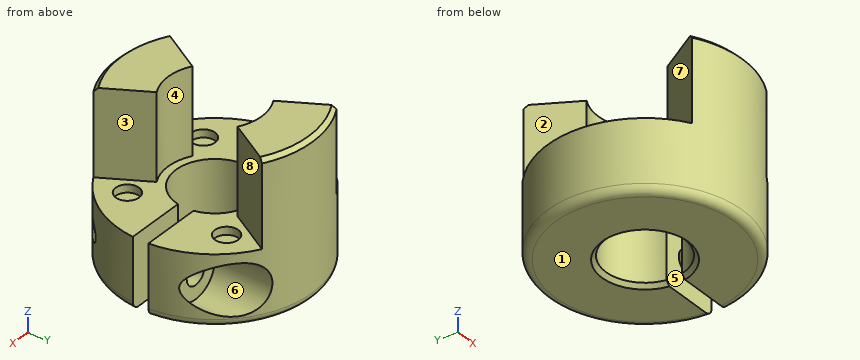
from build123d import *

# Parameters (mm, degrees)
ESBO_O1_R                 = 12.5
RESSALTO_EXTRUS_O1_DEPTH  = 20
CORTE_EXTRUS_O3_DEPTH     = 11
ESBO_O3_R                 = 5
CORTE_EXTRUS_O4_DEPTH     = 21
ESBO_O6_W                 = 12
ESBO_O6_H                 = 2
CORTE_EXTRUS_O5_DEPTH     = 10
CORTE_EXTRUS_O6_START     = -3
ESBO_O7_R                 = 3.25
CORTE_EXTRUS_O6_DEPTH     = 9.5
FURO_ROSCADO_DE_M3X0_51_D = 2.5
FILETE1_R                 = 1
ESBO_O10_R                = 1.5
CORTE_EXTRUS_O7_DEPTH     = 1
CHANFRO1_SIZE             = 0.5
CORTE_EXTRUS_O8_REACH     = 18.5
ESBO_O11_R                = 1.5
ESBO_O12_R                = 6
CORTE_EXTRUS_O9_DEPTH     = 11
PADR_OCIRCULAR1_COUNT     = 4
CHANFRO2_SIZE             = 0.5


with BuildPart() as part:
    # Esboço1 → Ressalto-extrusão1 (new body)
    with BuildSketch(Plane.XY):
        Circle(ESBO_O1_R)
    extrude(amount=RESSALTO_EXTRUS_O1_DEPTH)

    # Esboço2 → Corte-extrusão3 (cut)
    with BuildSketch(Plane.XY.offset(20)):
        with BuildLine():
            Line((0, 0), (6.25, 10.825317547))
            ThreePointArc((6.25, 10.825317547), (12.5, 0), (6.25, -10.825317547))
            Line((6.25, -10.825317547), (0, 0))
        make_face()
    corte_extrus_o3 = extrude(amount=-CORTE_EXTRUS_O3_DEPTH, mode=Mode.SUBTRACT)

    # Esboço3 → Corte-extrusão4 (cut, through all)
    with BuildSketch(Plane(origin=(0, 0, 0), x_dir=(-1, 0, 0), z_dir=(0, 0, -1))):
        Circle(ESBO_O3_R)
    extrude(amount=-CORTE_EXTRUS_O4_DEPTH, mode=Mode.SUBTRACT)

    # Espelhar1: Corte-extrusão3 across plane
    add(corte_extrus_o3.mirror(Plane(origin=(0, 0, 0), x_dir=(0, 0, 1), z_dir=(1, 0, 0))), mode=Mode.SUBTRACT)

    # Esboço6 → Corte-extrusão5 (cut, through all)
    with BuildSketch(Plane.XY.offset(9)):
        with Locations((7, 0)):
            Rectangle(ESBO_O6_W, ESBO_O6_H)
    extrude(amount=-CORTE_EXTRUS_O5_DEPTH, mode=Mode.SUBTRACT)

    # Esboço7 → Corte-extrusão6 (cut, through all)
    with BuildSketch(Plane.XZ.offset(-1).offset(CORTE_EXTRUS_O6_START)):
        with Locations((8.459935794, 4.5)):
            Circle(ESBO_O7_R)
    extrude(amount=-CORTE_EXTRUS_O6_DEPTH, mode=Mode.SUBTRACT)

    # Furo roscado de M3x0.51 (through all)
    with Locations(Plane(origin=(0, 4, 0), x_dir=(1, 0, 0), z_dir=(0, 1, 0))):
        with Locations((8.459935794, -4.5)):
            Hole(FURO_ROSCADO_DE_M3X0_51_D / 2)

    # Filete1
    filete1_edges = [part.edges().sort_by_distance(p)[0] for p in [
        (-12.5, 0, 0),
    ]]
    fillet(filete1_edges, radius=FILETE1_R)

    # Esboço10 → Corte-extrusão7 (cut)
    with BuildSketch(Plane.XY.offset(9)):
        with Locations((6.363961031, -6.363961031)):
            Circle(ESBO_O10_R)
    corte_extrus_o7 = extrude(amount=-CORTE_EXTRUS_O7_DEPTH, mode=Mode.SUBTRACT)

    # Chanfro1
    chanfro1_edges = [part.edges().sort_by_distance(p)[0] for p in [
        (0, -12.5, 20),
        (0, 12.5, 20),
    ]]
    chamfer(chanfro1_edges, length=CHANFRO1_SIZE)

    # Esboço11 → Corte-extrusão8 (cut, up to next)
    with BuildSketch(Plane(origin=(0, 4, 0), x_dir=(1, 0, 0), z_dir=(0, 1, 0)), mode=Mode.PRIVATE) as corte_extrus_o8_sk1:
        with Locations((8.459935794, -4.5)):
            Circle(ESBO_O11_R)
    corte_extrus_o8_tool1 = extrude(corte_extrus_o8_sk1.sketch, amount=-CORTE_EXTRUS_O8_REACH, mode=Mode.PRIVATE) & part.part
    add(corte_extrus_o8_tool1.solids().sort_by_distance((8.459936, 4, 4.5))[0], mode=Mode.SUBTRACT)

    # Esboço12 → Corte-extrusão9 (cut)
    with BuildSketch(Plane.XY.offset(20)):
        Circle(ESBO_O12_R)
    extrude(amount=-CORTE_EXTRUS_O9_DEPTH, mode=Mode.SUBTRACT)

    # PadrãoCircular1: Corte-extrusão7 ×4 about axis
    padr_ocircular1_axis = Axis((0, 0, 0), (0, 0, 1))
    for i in range(1, PADR_OCIRCULAR1_COUNT):
        add(corte_extrus_o7.rotate(padr_ocircular1_axis, i * 360 / PADR_OCIRCULAR1_COUNT), mode=Mode.SUBTRACT)

    # Chanfro2
    chanfro2_edges = [part.edges().sort_by_distance(p)[0] for p in [
        (-5, 0, 0),
    ]]
    chamfer(chanfro2_edges, length=CHANFRO2_SIZE)


solid = part.part
Geometry: final body of the model. Coordinates: model frame, mm. Face numbers are marked on the shaded views. A direction names the side the tool comes from. Give positions to 0.01 mm unless a question says otherwise; leave off trailing zeros. Order: outer loops, then holes, each group sorted by start corner. A loop starts at its lowest first (then second) coordinate and runs counter-clockwise, first axis right, second up. Notation, with made-up numbers: (32.5, -1.5) -> (91.5, -1.5) arc R17 ccw to (91.5, 2.5) -> close; hole circle Ø6 at (38.5, 3). An arc over 180 degrees is marked (long way). Answer as a JSON object with one key per item and string values.
Q1. Section C-C (z = 4.5). Output: boundary loops of the cut face in (x, y).
Entries:
{"outline": "(4.9, -1) arc R5 cw (long way) to (4.9, 1) -> (6.96, 1) -> (6.96, 4) -> (5.21, 4) -> (5.21, 11.36) arc R12.5 ccw (long way) to (7.21, -10.21) -> (7.21, -1) -> close; (9.71, -7.87) arc R12.5 ccw to (12.46, -1) -> (9.71, -1) -> close; (9.96, 1) -> (12.46, 1) arc R12.5 ccw to (11.71, 4.37) -> (11.71, 4) -> (9.96, 4) -> close"}
Q2. Material intervals for probe 1 along X at (y, z) = (-6.25, 4.5); probe 2 along X at (y, z) = (6.5, 8.5); probe 3 along X at (y, z) = (3.15, 4.5), sorted ascending.
Entries:
{"probe 1": "x = -10.83 to 7.21, 9.71 to 10.83", "probe 2": "x = -10.68 to -7.86, -4.87 to 4.87, 7.86 to 10.68", "probe 3": "x = -12.1 to -3.88, 3.88 to 6.96, 9.96 to 12.1"}
Q3. First-contact query: pin 1 (2.5 mm diameter, centred on x = -6.5, y = -7, fed in from +Z); pin 2 (2.5 mm diameter, centred on x = -6.36, y = -6.36, fed in from +Z); pin 3 (2.5 mm diameter, centred on x = 9.5, z = 5, fed in from +Y). Flat tips, straight axial feed; report the tip coordinate or a pass-through.
Entries:
{"pin 1": "stops at z = 9", "pin 2": "stops at z = 8", "pin 3": "stops at y = 4"}
Q4. Section B-B (x = 0). Output: boundary loops of the cut face in (y, z).
Entries:
{"outline": "(-12.5, 1) arc R1 ccw to (-11.5, 0) -> (-5.5, 0) -> (-5, 0.5) -> (-5, 9) -> (-6, 9) -> (-6, 20) -> (-12, 20) -> (-12.5, 19.5) -> close; (5, 0.5) -> (5.5, 0) -> (11.5, 0) arc R1 ccw to (12.5, 1) -> (12.5, 19.5) -> (12, 20) -> (6, 20) -> (6, 9) -> (5, 9) -> close"}
Q5. Draft query along X for the marked faces 1, 2, 3 and 4. Return one class per face: released by +X, released by -X, zero draft, split by the parting line, or undercut.
Entries:
{"face 1": "zero draft", "face 2": "released by -X", "face 3": "released by +X", "face 4": "undercut"}
Q6. Access query for the marked faces 5, 6, 7 and 8. Directions: +Z, -Z, +X, -X, +Y, -Y. A direction counts if a zero-diameter tool reaches every point of the face in a straight line with its end or side. Return the directions, or none.
Entries:
{"face 5": "+Z, -Z, +X", "face 6": "+Y", "face 7": "+Z, -X", "face 8": "+Z, +X"}
Q7. Section D-D (y = 0). Output: boundary loops of the cut face in (x, z), plus the area to 3 significant figures.
Entries:
{"outline": "(-12.5, 1) arc R1 ccw to (-11.5, 0) -> (-5.5, 0) -> (-5, 0.5) -> (-5, 9) -> (-12.5, 9) -> close", "area": "67.2 mm^2"}
Q8. Section A-A (z = 14.75). Output: boundary loops of the cut face in (x, y).
Entries:
{"outline": "(-6.25, -10.83) arc R12.5 ccw to (6.25, -10.83) -> (3, -5.2) arc R6 cw to (-3, -5.2) -> close; (-6.25, 10.83) -> (-3, 5.2) arc R6 cw to (3, 5.2) -> (6.25, 10.83) arc R12.5 ccw to start"}
